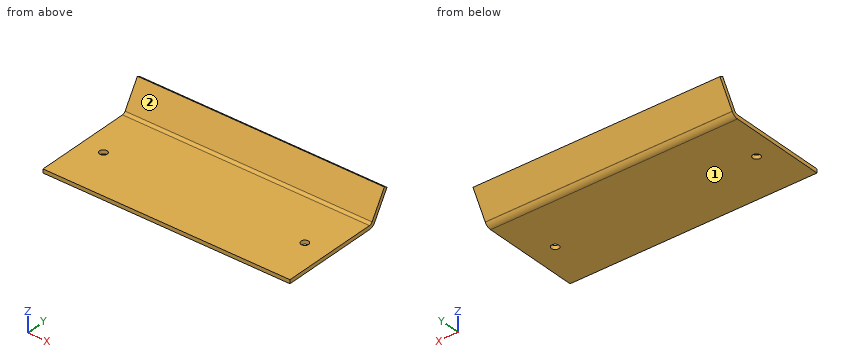
```python
from build123d import *

# Parameters (mm, degrees)
SKETCH1_W            = 260
SKETCH1_H            = 110
BASE_FLANGE1_DEPTH   = 4
EDGE_FLANGE1_START   = -153.944751381
EDGE_FLANGE1_DEPTH   = 260
EDGE_FLANGE1_2_DEPTH = 260
SKETCH11_R           = 4
CUT_EXTRUDE1_DEPTH   = 177.112626118


# Read off the part's stored shape, not the designer's step: Edge-Flange1
# Sheet-metal steps are written as plain solids
with BuildPart() as part:
    # Sketch1 → Base-Flange1 (new body)
    with BuildSketch(Plane.XY):
        with Locations((-23.944751381, -24.35359116)):
            Rectangle(SKETCH1_W, SKETCH1_H)
    extrude(amount=-BASE_FLANGE1_DEPTH)

    # Edge-Flange1 outline → Edge-Flange1 (cut)
    with BuildSketch(Plane.YZ.offset(EDGE_FLANGE1_START)):
        with BuildLine():
            Line((30.64640884, 0), (30.536111734, -0.179988518))
            ThreePointArc((30.536111734, -0.179988518), (27.623960351, -2.979968057), (23.714990419, -4))
            Line((23.714990419, -4), (30.64640884, -4))
            Line((30.64640884, -4), (30.64640884, 0))
        make_face()
    extrude(amount=EDGE_FLANGE1_DEPTH, mode=Mode.SUBTRACT)

    # Edge-Flange1 2 outline → Edge-Flange1 2 (add)
    with BuildSketch(Plane.YZ.offset(EDGE_FLANGE1_START)):
        with BuildLine():
            Line((23.714990419, 0), (30.64640884, 0))
            Line((30.64640884, 0), (46.482655452, 25.842405752))
            Line((46.482655452, 25.842405752), (43.072094795, 27.932400011))
            Line((43.072094795, 27.932400011), (27.125551077, 1.910005741))
            ThreePointArc((27.125551077, 1.910005741), (25.669475385, 0.510015972), (23.714990419, 0))
        make_face()
    extrude(amount=EDGE_FLANGE1_2_DEPTH)

    # Sketch11 → Cut-Extrude1 (cut, through all)
    with BuildSketch(Plane(origin=(0, 0, -4), x_dir=(-1, 0, 0), z_dir=(0, 0, -1))):
        with Locations((-81.055248619, -29.285009581)):
            Circle(SKETCH11_R)
        with Locations((130.944751381, -29.285009581)):
            Circle(SKETCH11_R)
    extrude(amount=-CUT_EXTRUDE1_DEPTH, mode=Mode.SUBTRACT)


solid = part.part
```
Could you check a few things on this model? Use its own coordinates, in mm. Face numbers are marked on the shaded views. Round coordinates to 2 decimals unless told otherwise and drop trailing zeros. Order: outer loops, then holes, each group sorted by start corner. A loop starts at its lowest first (then second) coordinate and runs counter-clockwise, first axis right, second up. Notation, with made-up numbers: (81, 68.5) -> (134, 68.5) arc R12 ccw to (134, 80.5) -> close; hole circle Ø6 at (48.25, -12). An arc over 180 degrees is marked (long way). One line per question, with ' | ' between items.
Q1. I'm going to push flat-ended pins straight in: pin 1 (1.5 mm diameter, centred on x = 8.5, y = -2, fed in from +Z); pin 2 (3 mm diameter, centred on x = -84.5, z = 16.5, fed in from -Y). Where does each tip first touch, or does it pass through?
Computed values:
pin 1: z = 0 | pin 2: y = 35.15
Q2. If we section it at B-B on y = -16: Write out the boundary of the cut face in (x, z), plus the area to 3 significant figures.
Computed values:
outline: (-153.94, -4) -> (106.06, -4) -> (106.06, 0) -> (-153.94, 0) -> close | area: 1,040 mm²
Q3. If I drill on line 1 (Z direction, x = 20, y = -35); line 2 (Y direction, x = -132.5, z = -2); line 3 (Y direction, x = -11, z = 23), over which ranges is the centre line in solid material (lowest first)? Write a range as from..to.
Computed values:
line 1: -4..0 | line 2: -79.35..-32.97, -25.6..29.01 | line 3: 40.05..44.74
Q4. If we section it at A-A on x = -131.5: Write out the boundary of the cut face in (y, z) (3 decimals), plus the area to 3 significant figures.
Computed values:
outline: (-79.354, -4) -> (-33.246, -4) -> (-33.246, 0) -> (-79.354, 0) -> close; (-25.324, -4) -> (23.715, -4) arc R8 ccw to (30.536, -0.18) -> (46.483, 25.842) -> (43.072, 27.932) -> (27.126, 1.91) arc R4 cw to (23.715, 0) -> (-25.324, 0) -> close | area: 527 mm²
Q5. If we section it at C-C on z = 4.5: Write out the boundary of the cut face in (x, y).
Computed values:
outline: (-153.94, 28.71) -> (106.06, 28.71) -> (106.06, 33.4) -> (-153.94, 33.4) -> close
Q6. We'd pull the mould along Z, two halves only. Please class the marked faces 1 and 2: released by +Z, released by -Z, zero draft, split by the parting line, or undercut.
Computed values:
face 1: released by -Z | face 2: released by +Z
